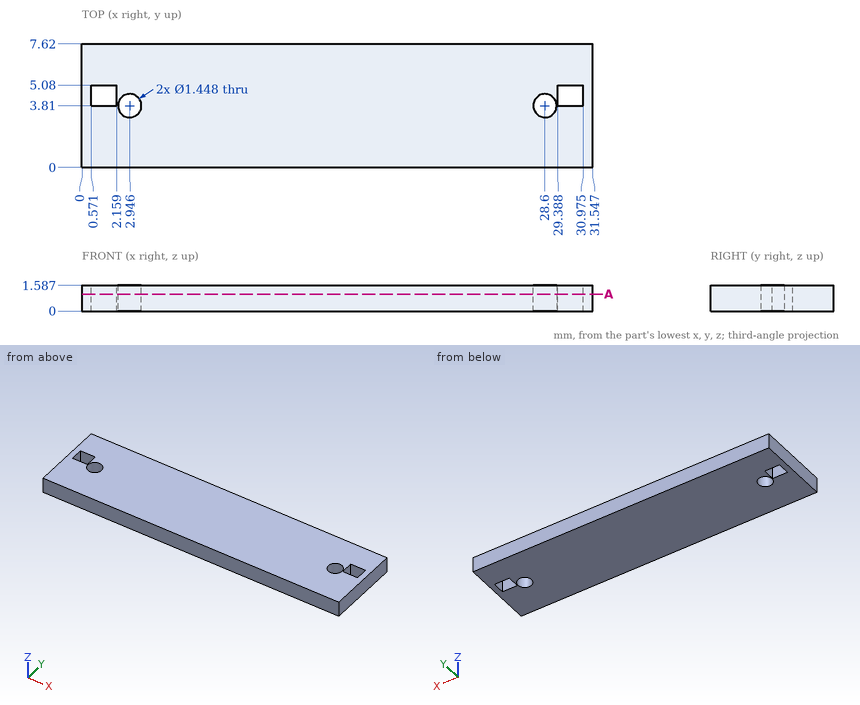
Geometry: see drawing. Coordinates: mm, zero at the bounding-box minimum. Coordinates: 2 decimals unless noted, no trailing zeros. Write each loop counter-clockwise with the first axis right and the second up, starting at its lowest first coordinate (ties: lowest second). Pieces come first, ordered by that corner, then holes.
1) Pin query (flat end, axial travel): pin 1 Ø0.8 at (x, z) = (1.5, 1) entering from -Y. Return the tip coordinate at first contact, or that it passes through.
2) Section A-A on z = 1.05. Output: boundary loops of the cut face in (x, y) (1 decimal), and give its area (3 significant figures).
3) Material intervals for line 1 along Y through (x, z) = (2, 1.3); line 2 along X through (y, z) = (4.25, 1.05) (1 decimal); line 3 along Y through (x, z) = (29, 0.65) (1 decimal), sorted ascending.
Check result:
1. pin 1: stops at y = 0
2. outline: (0, 0) - (31.5, 0) - (31.5, 7.6) - (0, 7.6) - close; hole (0.6, 3.8) - (2.2, 3.8) - (2.2, 5.1) - (0.6, 5.1) - close; hole circle Ø1.4 at (2.9, 3.8); hole circle Ø1.4 at (28.6, 3.8); hole (29.4, 3.8) - (31, 3.8) - (31, 5.1) - (29.4, 5.1) - close
2. area: 233 mm2
3. line 1: y = 0 to 3.81, 5.08 to 7.62
3. line 2: x = 0 to 0.6, 2.2 to 2.4, 3.5 to 28, 29.2 to 29.4, 31 to 31.5
3. line 3: y = 0 to 3.2, 4.4 to 7.6
